Can you work these out from the model? Positions are in its coordinate system, mm. A direction names the side the tool comes from. Coordinates: 2 decimals unless noted, no trailing zeros. Order: outer loops, then holes, each group sorted by start corner. A loop starts at its lowest first (then second) coordinate and runs counter-clockwise, first axis right, second up. Notation, with made-up numbers: M 61.5,-15.5 L 108.5,-15.5 A29 ccw 108.5,22.5 Z; hole C -9.75,-20 d2. An arc over 180 degrees is marked long. Answer as CSV lines item,"result". Start each with the question number.
1. If we section it at B-B (x = -1): List the corners of the cut face in (y, z) for me.
2. If we section it at C-C (x = -16.5): List the corners of the cut face in (y, z) for me.
3. I need wall thicknesses on line 1 along Y through (x, z) = (0, 10); line 2 along Z through (x, y) = (-21, -17.5); line 3 along X through (y, z) = (0.5, 3). Which ranges of each line are inside material? Lowest first, please. Write a range as from..to.
4. If we mould it in two halves opening along Y, with no side actions, what happens to faces 1 (the face through (0, 8, 0)), 2 (the face through (12.114, -2.662, 6.439)), 3 (the face through (-18.157, -24.239, 6.439))? For each: released by +Y, released by -Y, zero draft, split by the parting line, or undercut.
5. Will these pins go through, and if not, where does the flat tip stop? pin 1 (8 mm diameter, centred on x = -9, y = -14.5, fed in from +Z); pin 2 (10 mm diameter, centred on y = 22.5, z = 34.5, fed in from -X).
6. If we section it at D-D (z = 31): List the corners of the cut face in (x, y) for me, plus the area to 3 significant figures.
7. On a 3-axis mill with a long thin cutter (end or side, diameter ignored), from which of +Z, -Z, +X, -X, +Y, -Y can I reach the whole of each face in a straight line? I mean faces 4 (the face through (0, 8, 12.7)), 5 (the face through (-12.7, 25, 32)), 6 (the face through (-25.4, 12, 6)). Say none if no direction works.
8. If we section it at A-A (y = -10.5): List the corners of the cut face in (x, z) for me, plus the area to 3 significant figures.
```python
from build123d import *

# Parameters (mm, degrees)
F0_W     = 50.8
F0_H     = 63.754
F1_DEPTH = 12.7
F2_W     = 50.8
F2_H     = 13.0302
F3_DEPTH = 38.1
F4_W     = 12.7
F4_H     = 13.0302
F5_DEPTH = 12.7
F6_R     = 25.39999
F7_R     = 12.7
F8_DEPTH = 12.701


# Not quite as in the source:
# - a fillet or chamfer is up to 0.001 mm smaller than in the source, because OpenCascade refuses the exact size


with BuildPart() as f1:
    # F0 (on Top) → F1 (new body)
    with BuildSketch(Plane.XY):
        Rectangle(F0_W, F0_H)
    extrude(amount=F1_DEPTH)

    # F2 (on Top) → F3 (join)
    with BuildSketch(Plane.XY):
        with Locations((1.8626e-06, 25.3619)):
            Rectangle(F2_W, F2_H)
    extrude(amount=F3_DEPTH)

    # F4 (on face) → F5 (cut)
    with BuildSketch(Plane.XY.offset(38.1)):
        with Locations((-19.0499981374, 25.3619)):
            Rectangle(F4_W, F4_H)
    extrude(amount=-F5_DEPTH, mode=Mode.SUBTRACT)

    # F6 (radius 25.4 in the source; OpenCascade refuses exactly that, so slightly less here)
    f6_edges = [f1.edges().sort_by_distance(p)[0] for p in [
        (-25.4, -31.877, 6.35),
        (25.4, -31.877, 6.35),
    ]]
    fillet(f6_edges, radius=F6_R)

    # F7 (on face) → F8 (cut, through all)
    with BuildSketch(Plane.XY.offset(12.7)):
        with Locations((0, -6.477)):
            Circle(F7_R)
    extrude(amount=-F8_DEPTH, mode=Mode.SUBTRACT)


solid = f1.part
```
Solved:
1,outline,"M -31.86,0 L -19.14,0 L -19.14,12.7 L -31.86,12.7 Z; M 6.18,0 L 31.88,0 L 31.88,38.1 L 18.85,38.1 L 18.85,12.7 L 6.18,12.7 Z"
2,outline,"M -25.79,0 L 31.88,0 L 31.88,25.4 L 18.85,25.4 L 18.85,12.7 L -25.79,12.7 Z"
3,line 1,"-31.88..-19.18, 6.22..31.88"
3,line 2,"0..12.7"
3,line 3,"-25.4..-10.61, 10.61..25.4"
4,face 1,"zero draft"
4,face 2,"undercut"
4,face 3,"released by -Y"
5,pin 1,"z = 12.7"
5,pin 2,"x = -12.7"
6,outline,"M -12.7,18.85 L 25.4,18.85 L 25.4,31.88 L -12.7,31.88 Z"
6,area,"496 mm²"
7,face 4,"+Z, +X, -X, -Y"
7,face 5,"+Z, -X, +Y, -Y"
7,face 6,"+Z, -Z, -X, +Y, -Y"
8,outline,"M -25.08,0 L -12.05,0 L -12.05,12.7 L -25.08,12.7 Z; M 12.05,0 L 25.08,0 L 25.08,12.7 L 12.05,12.7 Z"
8,area,"331 mm²"
